Geometry: final body of the model. Coordinates: model frame, mm. A direction names the side the tool comes from. Round coordinates to 2 decimals unless told otherwise and drop trailing zeros. Order: outer loops, then holes, each group sorted by start corner. A loop starts at its lowest first (then second) coordinate and runs counter-clockwise, first axis right, second up. Notation, with made-up numbers: (-12.75, 67.25) -> (8.25, 67.25) arc R26 cw to (8.25, 97.25) -> close; hole circle Ø6 at (85.25, 25.25). An arc over 180 degrees is marked (long way). Put each result on its own line as item: value.
```python
from build123d import *

# Parameters (mm, degrees)
F0_W     = 772
F0_H     = 640
F1_DEPTH = 2
F2_W     = 0.25
F2_H     = 119.9
F3_DEPTH = 25
F4_DEPTH = 25
F2_W_2   = 119.9
F2_H_2   = 0.2
F2_W_3   = 0.2
F2_H_3   = 399.8
F5_DEPTH = 25
F2_W_4   = 64.7
F6_DEPTH = 25
F2_W_5   = 55
F7_DEPTH = 25
F2_H_4   = 49.5626640439
F8_DEPTH = 25
F2_H_5   = 199.6
F2_W_6   = 9.8
F2_H_6   = 30.4373359561
F2_W_7   = 10
F2_H_7   = 29.8
F9_DEPTH = 25


# Not quite as in the source:
# - a feature names something its author has since deleted; it is built from what else it names


with BuildPart() as f1:
    # F0 (on Top) → F1 (new body)
    with BuildSketch(Plane.XY):
        with Locations((386, 320)):
            Rectangle(F0_W, F0_H)
    extrude(amount=F1_DEPTH)

    # F2 (on face) → F3 (join)
    with BuildSketch(Plane.XY.offset(2)):
        with Locations((651.975, 580.05)):
            Rectangle(F2_W, F2_H)
        with Locations((120.025, 580.05)):
            Rectangle(F2_W, F2_H)
        Polygon((120.1, 119.9), (119.9, 119.9), (119.9, 0), (120.15, 0), (120.15, 119.9), align=None)
        Polygon((652.1, 119.9), (651.9, 119.9), (651.85, 119.9), (651.85, 0), (652.1, 0), align=None)
    extrude(amount=-F3_DEPTH)

    # F2 (on face) → F4 (join)
    with BuildSketch(Plane.XY.offset(2)):
        Polygon((119.9, 520.1), (0, 520.1), (0, 519.9), (55, 519.9), (55.2, 519.9), (119.9, 519.9), align=None)
        Polygon((651.85, 520.1), (120.15, 520.1), (120.15, 519.9), (651.9, 519.9), (652.1, 519.9), (652.1, 520.1), align=None)
    extrude(amount=F4_DEPTH)

    # F2 (on face) → F5 (join)
    with BuildSketch(Plane.XY.offset(2)):
        with Locations((712.05, 520)):
            Rectangle(F2_W_2, F2_H_2)
        with Locations((652, 320)):
            Rectangle(F2_W_3, F2_H_3)
    extrude(amount=F5_DEPTH)

    # F2 (on face) → F6 (join)
    with BuildSketch(Plane.XY.offset(2)):
        with Locations((712.05, 120)):
            Rectangle(F2_W_2, F2_H_2)
        Polygon((651.9, 120.1), (120.1, 120.1), (120.1, 119.9), (120.15, 119.9), (651.85, 119.9), (651.9, 119.9), align=None)
        with Locations((652, 120)):
            Rectangle(F2_W_3, F2_H_2)
        with Locations((87.55, 120)):
            Rectangle(F2_W_4, F2_H_2)
        with Locations((120, 120)):
            Rectangle(F2_W_3, F2_H_2)
    extrude(amount=F6_DEPTH)

    # F2 (on face) → F7 (join)
    with BuildSketch(Plane.XY.offset(2)):
        with Locations((27.5, 120)):
            Rectangle(F2_W_5, F2_H_2)
    extrude(amount=F7_DEPTH)

    # F2 (on face) → F8 (join)
    with BuildSketch(Plane.XY.offset(2)):
        with Locations((55.1, 175.318667978)):
            Rectangle(F2_W_3, F2_H_4)
    extrude(amount=F8_DEPTH)

    # F2 (on face) → F9 (join)
    with BuildSketch(Plane.XY.offset(2)):
        Polygon((120.15, 520.1), (119.9, 520.1), (119.9, 519.9), (120.1, 519.9), (120.15, 519.9), align=None)
        with Locations((120, 320)):
            Rectangle(F2_W_3, F2_H_3)
        with Locations((55.1, 420.1)):
            Rectangle(F2_W_3, F2_H_5)
        with Locations((55.1, 320.2)):
            Rectangle(F2_W_3, F2_H_2)
        with Locations((50.1, 320.2)):
            Rectangle(F2_W_6, F2_H_2)
        with Locations((55.1, 135.318667978)):
            Rectangle(F2_W_3, F2_H_6)
        with Locations((55.1, 120)):
            Rectangle(F2_W_3, F2_H_2)
        with Locations((60.2, 320.2)):
            Rectangle(F2_W_7, F2_H_2)
        with Locations((55.1, 305.2)):
            Rectangle(F2_W_3, F2_H_7)
        with Locations((55.1, 175.318667978)):
            Rectangle(F2_W_3, F2_H_4)
        with Locations((55.1, 290.2)):
            Rectangle(F2_W_3, F2_H_2)
        with Locations((50.1, 290.2)):
            Rectangle(F2_W_6, F2_H_2)
        with Locations((50.1, 200.2)):
            Rectangle(F2_W_6, F2_H_2)
        with Locations((55.1, 200.2)):
            Rectangle(F2_W_3, F2_H_2)
        with Locations((60.2, 290.2)):
            Rectangle(F2_W_7, F2_H_2)
        with Locations((60.2, 200.2)):
            Rectangle(F2_W_7, F2_H_2)
        with Locations((55.1, 275.2)):
            Rectangle(F2_W_3, F2_H_7)
        with Locations((55.1, 215.2)):
            Rectangle(F2_W_3, F2_H_7)
        with Locations((55.1, 260.2)):
            Rectangle(F2_W_3, F2_H_2)
        with Locations((50.1, 260.2)):
            Rectangle(F2_W_6, F2_H_2)
        with Locations((50.1, 230.2)):
            Rectangle(F2_W_6, F2_H_2)
        with Locations((55.1, 230.2)):
            Rectangle(F2_W_3, F2_H_2)
        with Locations((60.2, 260.2)):
            Rectangle(F2_W_7, F2_H_2)
        with Locations((60.2, 230.2)):
            Rectangle(F2_W_7, F2_H_2)
        with Locations((55.1, 245.2)):
            Rectangle(F2_W_3, F2_H_7)
    extrude(amount=F9_DEPTH)


solid = f1.part
```
1. Cut plane D-D on y = 99.5. Return loops of the section in (x, z).
Ans:
outline: (0, 0) -> (119.9, 0) -> (119.9, -23) -> (120.15, -23) -> (120.15, 0) -> (651.85, 0) -> (651.85, -23) -> (652.1, -23) -> (652.1, 0) -> (772, 0) -> (772, 2) -> (0, 2) -> close
2. Cut plane C-C on x = 300. Return loops of the section in (y, z), and give its area (3 significant figures).
Ans:
outline: (0, 0) -> (640, 0) -> (640, 2) -> (520.1, 2) -> (520.1, 27) -> (519.9, 27) -> (519.9, 2) -> (120.1, 2) -> (120.1, 27) -> (119.9, 27) -> (119.9, 2) -> (0, 2) -> close
area: 1,290 mm²
3. Material intervals for probe 1 along X at (y, z) = (182.5, 15); probe 2 along X at (y, z) = (75, -9); probe 3 along Y at (x, z) = (645, 12), sorted ascending.
Ans:
probe 1: 55 to 55.2, 119.9 to 120.1, 651.9 to 652.1
probe 2: 119.9 to 120.15, 651.85 to 652.1
probe 3: 119.9 to 120.1, 519.9 to 520.1
4. Cut plane B-B on y = 361. Return loops of the section in (x, z).
Ans:
outline: (0, 0) -> (772, 0) -> (772, 2) -> (652.1, 2) -> (652.1, 27) -> (651.9, 27) -> (651.9, 2) -> (120.1, 2) -> (120.1, 27) -> (119.9, 27) -> (119.9, 2) -> (55.2, 2) -> (55.2, 27) -> (55, 27) -> (55, 2) -> (0, 2) -> close
5. Set-up query: faces 1 (the face through (55, 215, 14)), 2 (the face through (381, 61, 2)), 3 (the face through (391, 520.1, 14)), 4 (the face through (87, 519.9, 14)). Return all of +Z, -Z, +X, -X, +Y, -Y with unobstructed straight access to the full face (end or side cutting, diameter ignored); none if empty.
Ans:
face 1: +Z, -X
face 2: +Z, +X, -X, -Y
face 3: +Z, +X, -X, +Y
face 4: +Z
6. Draft query along X for faces 5 (the face through (772, 318.5, 0.4)), 6 (the face through (713, 120.1, 14)), 7 (the face through (382, 519.9, 14)). Return one class per face: +X half, -X half, draft (parallel to the pull), parting line (faces both ways), or undercut.
Ans:
face 5: +X half
face 6: draft
face 7: undercut
7. Contact query for flat-ended pins moving along their axis: P1, Ø3, axis at x = 49.5, z = 12.5, coming from the -Y side; P2, Ø11, axis at x = 49.5, z = 10.5, coming from the +Y side; P3, Ø7.5, axis at y = 359, z = 15, coming from the +X side. Output: stop coordinate, or through.
Ans:
P1: y = 119.9
P2: y = 520.1
P3: x = 652.1
8. Cut plane A-A on z = -9.5. Return loops of the section in (x, y).
Ans:
outline: (119.9, 0) -> (120.15, 0) -> (120.15, 119.9) -> (119.9, 119.9) -> close; (119.9, 520.1) -> (120.15, 520.1) -> (120.15, 640) -> (119.9, 640) -> close; (651.85, 0) -> (652.1, 0) -> (652.1, 119.9) -> (651.85, 119.9) -> close; (651.85, 520.1) -> (652.1, 520.1) -> (652.1, 640) -> (651.85, 640) -> close
